Solid Edge part; units mm, degrees
sketch "Sketch1" plane through (0, 0, 0) normal (0, 0, 1) x (1, 0, 0)
  circle A0 centre (0, 0) radius 14
extrude "Protrusion1" add sketch "Sketch1" along normal blind 20
sketch "Sketch2" plane through (0, 0, 0) normal (0, 0, 1) x (1, 0, 0)
  line L0 (-7.5, -18) -> (7.5, -18)
  line L1 (7.5, -18) -> (7.5, -8.1391)
  line L2 (7.5, -8.1391) -> (-7.5, -8.1391)
  line L3 (-7.5, -8.1391) -> (-7.5, -18)
  dimension "D1" = 7.5
extrude "ExtrudedProtrusion_2" add sketch "Sketch2" along normal blind 17
sketch "Sketch3" plane through (0, 0, 0) normal (0, 0, 1) x (1, 0, 0)
  circle A0 centre (-17.5, 0) radius 2
  circle A1 centre (17.5, 0) radius 2
  line L0 (-17.5, 3.5) -> (17.5, 3.5)
  line L1 (-17.5, -3.5) -> (17.5, -3.5)
  arc A2 (-17.5, -3.5) -> (-17.5, 3.5) centre (-17.5, 0) cw
  arc A3 (17.5, 3.5) -> (17.5, -3.5) centre (17.5, 0) cw
extrude "ExtrudedProtrusion_3" add sketch "Sketch3" along normal blind 1
sketch "Sketch4" plane through (0, -2, 0) normal (0, 0, -1) x (1, 0, 0)
  circle A0 centre (0, -10) radius 4.5
extrude "ExtrudedProtrusion_4" add sketch "Sketch4" along normal blind 1.5
sketch "Sketch5" plane through (0, -2, 0) normal (0, 0, -1) x (1, 0, 0)
  circle A0 centre (0, -10) radius 2.5
extrude "ExtrudedProtrusion_5" add sketch "Sketch5" along normal blind 10
chamfer "Letörés_1" distance 0.5 angle 45 1 edges at (-2.5, 8, -10)
sketch "Sketch6" plane through (0, 8, -10) normal (0, 0, -1) x (1, 0, 0)
  line L0 (-7.2706, -6.0348) -> (6.189, -6.0348)
  line L1 (6.189, -6.0348) -> (6.189, -1.5)
  line L2 (6.189, -1.5) -> (-7.2706, -1.5)
  line L3 (-7.2706, -1.5) -> (-7.2706, -6.0348)
  line L4 (-5.1689, 1.5) -> (6.5499, 1.5)
  line L5 (6.5499, 1.5) -> (6.5499, 5.1107)
  line L6 (6.5499, 5.1107) -> (-5.1689, 5.1107)
  line L7 (-5.1689, 5.1107) -> (-5.1689, 1.5)
extrude "ExtrudedCutout_1" cut sketch "Sketch6" against normal blind 6
Here's how the part is built. I have some questions about the finished solid (model axes, mm). A direction names the side the tool comes from. Give positions to 0.01 mm unless a question says otherwise; leave off trailing zeros. Write each loop counter-clockwise with the first axis right and the second up, starting at its lowest first coordinate (ties: lowest second). Pieces come first, ordered by that corner, then holes. Notation, with made-up numbers: M 19,-20.5 L 54,-20.5 A21 ccw 54,2.5 Z; hole C 68.5,-30.75 d8. An arc over 180 degrees is marked long. Put each result on its own line as item: value. Start each with the question number.
Item 1: Will these pins go through, and if not, where does the flat tip stop? pin 1 (8 mm diameter, centred on y = -14, z = 11, fed in from -X); pin 2 (10 mm diameter, centred on y = -6.5, z = 13, fed in from +X); pin 3 (3 mm diameter, centred on y = -16, z = 7.5, fed in from -X); pin 4 (3.5 mm diameter, centred on x = 17.5, y = 0, fed in from -Z).
Item 2: On a 3-axis mill with a long thin cutter (end or side, diameter ignored), from which of +Z, -Z, +X, -X, +Y, -Y can I reach the whole of each face in a straight line? I mean faces 5 (the flat face through (7.5, -15, 8)), 6 (the flat face through (0, 10, -4)), 7 (the flat face through (15.5, 3.5, 0.5)), 8 (the cylindrical face through (-0.59, 12.46, -0.74)), 9 (the flat face through (-15.6, 3.5, 0.5)). Say none if no direction works.
Item 3: If we section it at B-B, the plane y = 1: Write out the boundary of the cut face in (x, z).
Item 4: I need wall thicknesses on L1, parallel to Y at x = 17.5, z = 0.65; L2, parallel to Z at x = 4, y = -11; L3, parallel to X at y = 0, z = 8.5. Which ranges of each line are inside material? Lowest first, please. Write a range as from..to.
Item 5: If we section it at C-C, the plane z = 2.25: Write out the boundary of the cut face in (x, y).
Item 6: If we section it at A-A, the plane x = 0: Write out the boundary of the cut face in (y, z), then the cut area to 3 significant figures.
Item 7: If we section it at D-D, the plane y = 8: Write out the boundary of the cut face in (x, z).
Item 8: Thinking about a two-plate mould opening in Y: for faces 1 (the cylindrical face through (2.385, 8.751, -4.555)), 2 (the flat face through (0, 6, -4)), 3 (the flat face through (0, 6.5, -7)), 4 (the cylindrical face through (-19.1, 1.2, 0.5)), which applies, +Y half, -Y half, draft (parallel to the pull), parting line (faces both ways), or undercut?
Values:
1. pin 1: x = -9.8
1. pin 2: x = 13.92
1. pin 3: x = -7.5
1. pin 4: through
2. face 5: +Z, -Z, +X, -Y
2. face 6: -Z, +X, -X, +Y
2. face 7: +Z, -Z, +X, +Y
2. face 8: -Z
2. face 9: +Z, -Z, -X, +Y
3. outline: M -20.85,0 L -19.23,0 L -19.23,1 L -20.85,1 Z; M -15.77,0 L 15.77,0 L 15.77,1 L 13.96,1 L 13.96,20 L -13.96,20 L -13.96,1 L -15.77,1 Z; M 19.23,0 L 20.85,0 L 20.85,1 L 19.23,1 Z
4. L1: -3.5..-2, 2..3.5
4. L2: 0..20
4. L3: -14..14
5. outline: M -7.5,-18 L 7.5,-18 L 7.5,-11.82 A14 ccw long -7.5,-11.82 Z
6. outline: M -18,0 L 3.5,0 L 3.5,-1.5 L 5.5,-1.5 L 5.5,-4 L 6.5,-4 L 6.5,-10 L 9.5,-10 L 9.5,-4 L 10.5,-4 L 10.5,-1.5 L 12.5,-1.5 L 12.5,0 L 14,0 L 14,20 L -14,20 L -14,17 L -18,17 Z
6. area: 672 mm²
7. outline: M -11.49,0 L -4.5,0 L -4.5,-1.5 L -2.5,-1.5 L -2.5,-9.5 L -2,-10 L 2,-10 L 2.5,-9.5 L 2.5,-1.5 L 4.5,-1.5 L 4.5,0 L 11.49,0 L 11.49,20 L -11.49,20 Z
8. face 1: parting line
8. face 2: draft
8. face 3: -Y half
8. face 4: undercut
